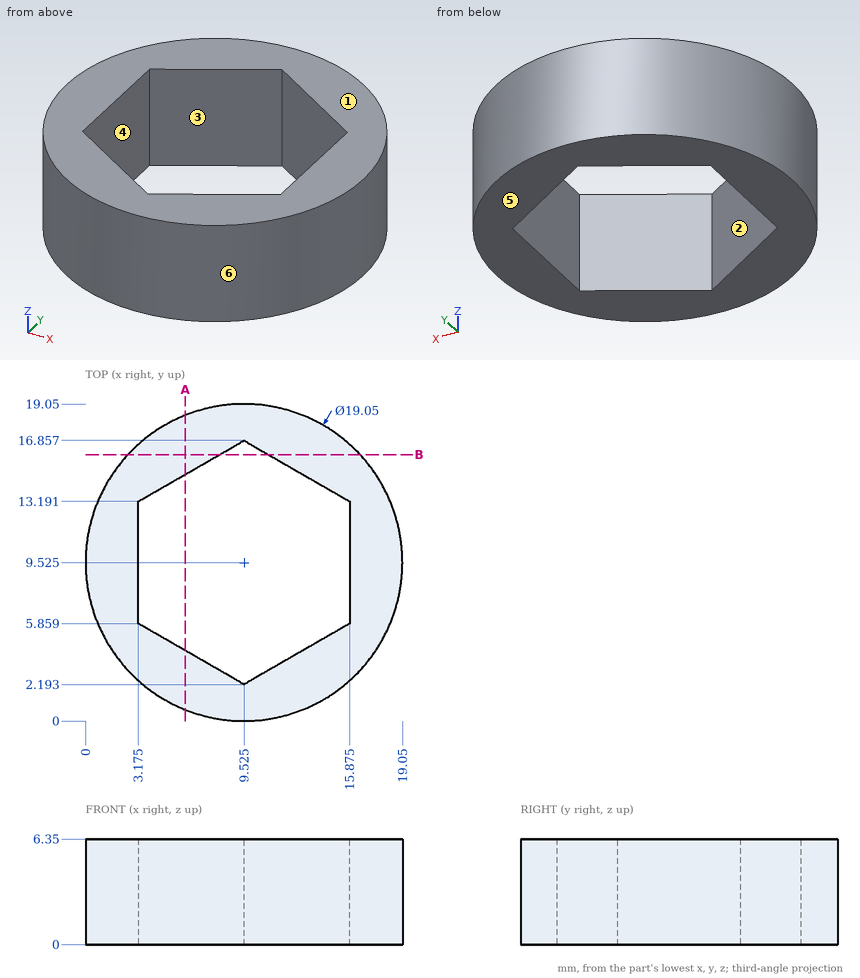
Design review of the part shown in the three views and the two pictorial views. Dimensions are in mm from the part's minimum x, y and z. A direction names the side the tool comes from. Round coordinates to 2 decimals unless told otherwise and drop trailing zeros. Loops run counter-clockwise (first coordinate to the right, second up) from the corner with the lowest first, then second, coordinate; pieces in that order, holes last.
1) Consider section A-A on x = 6. State the section outline as (y, z) points.
Values follow:
outline: (0.68, 0) - (4.23, 0) - (4.23, 6.35) - (0.68, 6.35) - close; (14.82, 0) - (18.37, 0) - (18.37, 6.35) - (14.82, 6.35) - close
2) Wall thickness on line 1 along X through (y, z) = (16.25, 4) (1 decimal); line 2 along X through (y, z) = (5.75, 6) (1 decimal); line 3 along Y through (x, z) = (13.25, 3.25): over which ranges is each line inside the solid? List them lowest first.
Values follow:
line 1: x = 2.8 to 8.5, 10.6 to 16.3
line 2: x = 0.8 to 3.4, 15.7 to 18.3
line 3: y = 0.76 to 4.34, 14.71 to 18.29
3) The part is to be moulded in two halves that separate along Y. For the marked faces 3, 4, 5 and 6, say which applies: pulls with the +Y half, pulls with the -Y half, needs draft (parallel to the pull), parting line crosses it, or undercut.
Values follow:
face 3: undercut
face 4: undercut
face 5: needs draft
face 6: parting line crosses it
4) Clearance check with flat-ended pins moving along their axes: P1, Ø6, axis at x = 5.5, y = 6.5, coming from the +Z side; P2, Ø2, axis at x = 16, z = 3.5, coming from the -Y side; P3, Ø2, axis at x = 3.5, z = 2.5, coming from the -Y side. State where each tip first meets the part, or that it passes through.
Values follow:
P1: stops at z = 6.35
P2: stops at y = 1.73
P3: stops at y = 1.43
5) Consider section B-B on y = 16. State the section outline as (x, z) points.
Values follow:
outline: (2.54, 0) - (8.04, 0) - (8.04, 6.35) - (2.54, 6.35) - close; (11.01, 0) - (16.51, 0) - (16.51, 6.35) - (11.01, 6.35) - close
6) Tool access review of the marked faces 1 and 2: name each direction out of +Z, -Z, +X, -X, +Y, -Y from which nothing blocks a thin tool from reaching the whole face with its end or side.
Values follow:
face 1: +Z, +X, -X, +Y, -Y
face 2: +Z, -Z
